```python
from build123d import *

# Parameters (mm, degrees)
SKETCH_1_R          = 18.5
EXTRUDE_1_DEPTH     = 26.5
SKETCH_2_R          = 16.25
EXTRUDE_2_DEPTH     = 21.9
SKETCH_3_R          = 6
EXTRUDE_3_DEPTH     = 6
SKETCH_4_R          = 3
EXTRUDE_4_DEPTH     = 15
CUT_EXTRUDE_START   = -12
CUT_EXTRUDE_1_DEPTH = 12
FILLET_1_R          = 0.5
SKETCH_6_R          = 1.5
CUT_EXTRUDE_2_DEPTH = 3


with BuildPart() as part:
    # 草图1 → 凸台-拉伸1 (new body)
    with BuildSketch(Plane(origin=(0, 0, 0), x_dir=(1, 0, 0), z_dir=(0, 1, 0))):
        with Locations(Location((0, 0, 0), (0, 0, 270))):
            Circle(SKETCH_1_R)
    extrude(amount=EXTRUDE_1_DEPTH)

    # 草图2 → 凸台-拉伸2 (add)
    with BuildSketch(Plane(origin=(0, 26.5, 0), x_dir=(1, 0, 0), z_dir=(0, 1, 0))):
        with Locations(Location((0, 0, 0), (0, 0, 270))):
            Circle(SKETCH_2_R)
    extrude(amount=EXTRUDE_2_DEPTH)

    # 草图3 → 凸台-拉伸3 (add)
    with BuildSketch(Plane.XZ):
        with Locations(Location((-7, 0, 0), (0, 0, 90))):
            Circle(SKETCH_3_R)
    extrude(amount=EXTRUDE_3_DEPTH)

    # 草图4 → 凸台-拉伸4 (add)
    with BuildSketch(Plane.XZ.offset(6)):
        with Locations(Location((-7, 0, 0), (0, 0, 270))):
            Circle(SKETCH_4_R)
    extrude(amount=EXTRUDE_4_DEPTH)

    # 草图5 → 切除-拉伸1 (cut)
    with BuildSketch(Plane.XZ.offset(21).offset(CUT_EXTRUDE_START)):
        with BuildLine():
            Line((-9.4, -1.8), (-9.4, 1.8))
            ThreePointArc((-9.4, 1.8), (-10, 0), (-9.4, -1.8))
        make_face()
    extrude(amount=CUT_EXTRUDE_1_DEPTH, mode=Mode.SUBTRACT)

    # 圆角1
    fillet_1_edges = [part.edges().sort_by_distance(p)[0] for p in [
        (0, 0, -18.5),
        (0, 26.5, -18.5),
        (0, 48.4, -16.25),
    ]]
    fillet(fillet_1_edges, radius=FILLET_1_R)

    # 草图6 → 切除-拉伸2 (cut)
    with BuildSketch(Plane.XZ):
        with Locations(Location((0, -15.5, 0), (0, 0, 270))):
            Circle(SKETCH_6_R)
        with Locations(Location((-13.423393759, -7.75, 0), (0, 0, 270))):
            Circle(SKETCH_6_R)
        with Locations(Location((-13.423393759, 7.75, 0), (0, 0, 270))):
            Circle(SKETCH_6_R)
        with Locations(Location((0, 15.5, 0), (0, 0, 270))):
            Circle(SKETCH_6_R)
        with Locations(Location((13.423393759, 7.75, 0), (0, 0, 270))):
            Circle(SKETCH_6_R)
        with Locations(Location((13.423393759, -7.75, 0), (0, 0, 270))):
            Circle(SKETCH_6_R)
    extrude(amount=-CUT_EXTRUDE_2_DEPTH, mode=Mode.SUBTRACT)


solid = part.part
```
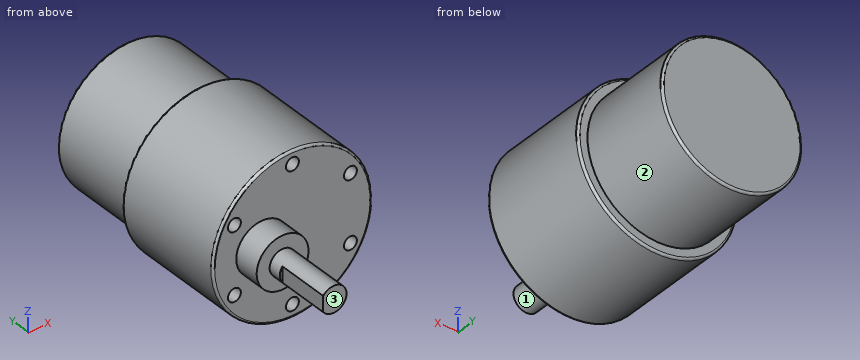
Check sheet for the modelled part. Datum: model origin and axes. Units: mm. Face numbers are marked on the shaded views. A direction names the side the tool comes from. Give positions to 0.01 mm unless a question says otherwise; leave off trailing zeros. Order: outer loops, then holes, each group sorted by start corner. A loop starts at its lowest first (then second) coordinate and runs counter-clockwise, first axis right, second up. Notation, with made-up numbers: M 81.5,-1 L 106.5,-1 A24 ccw 106.5,36 Z; hole C -2.75,7 d7. An arc over 180 degrees is marked long. Answer in a Markdown table with one row per item. Add a question column.
Q1. Gauge pin test, flat ends, axial feed: pin 1 Ø2.5 at (x, z) = (13, 7.5) entering from -Y; pin 2 Ø1.5 at (x, y) = (-6.5, 20.5) entering from -Z; pin 3 Ø1.5 at (x, z) = (-14, 8) entering from -Y; pin 4 Ø4 at (y, z) = (-3.5, -13.5) entering from -X. Record the tip position at first contact, or that the pin passes through.
Q2. Sectioned sample at B-B, the plane y = -1.5. Record the boundary of the cut face in (x, z).
Q3. Access from +Z, -Z, +X, -X, +Y, -Y to the whole of each face (thin tool, end or side, straight path). Record for the marked faces 1, 2 and 3.
Q4. Sectioned sample at C-C, the plane y = 35. Record the boundary of the cut face in (x, z).
Q5. Sectioned sample at A-A, the plane z = 0. Record the boundary of the cut face in (x, y).
Q6. Thickness scan on L1, parallel to X at y = 1.85, z = 7.75; L2, parallel to Y at x = 4, z = 4; L3, parallel to X at y = 1.15, z = -15.5. Record the ranges inside material, lowest first.
Verdict:
| question | item | result |
|---|---|---|
| 1 | pin 1 | y = 0 |
| 1 | pin 2 | z = -17.58 |
| 1 | pin 3 | y = 3 |
| 1 | pin 4 | through |
| 2 | outline | C -7,0 d12 |
| 3 | face 1 | -Y |
| 3 | face 2 | +Y |
| 3 | face 3 | +Z, -Z, +X, -X, -Y |
| 4 | outline | C 0,0 d32.5 |
| 5 | outline | M -18.5,0.5 A0.5 ccw -18,0 L -13,0 L -13,-6 L -10,-6 L -10,-9 L -9.4,-9 L -9.4,-21 L -4,-21 L -4,-6 L -1,-6 L -1,0 L 18,0 A0.5 ccw 18.5,0.5 L 18.5,26 A0.5 ccw 18,26.5 L 16.25,26.5 L 16.25,47.9 A0.5 ccw 15.75,48.4 L -15.75,48.4 A0.5 ccw -16.25,47.9 L -16.25,26.5 L -18,26.5 A0.5 ccw -18.5,26 Z |
| 6 | L1 | -16.8 to -14.92, -11.92 to 11.92, 14.92 to 16.8 |
| 6 | L2 | 0 to 48.4 |
| 6 | L3 | -10.1 to -1.5, 1.5 to 10.1 |
